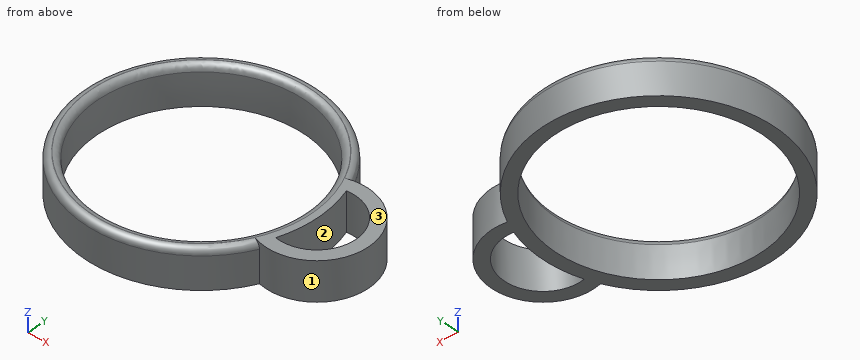
```python
from build123d import *

# Parameters (mm, degrees)
F4_DEPTH = 1.5
F5_DEPTH = 1.5
F6_R     = 0.5


with BuildPart() as f2:
    # F1 (on Front) → F2 (revolve)
    with BuildSketch(Plane.XZ):
        with BuildLine():
            Line((-8.0375234668, 1.5), (-9.0375234668, 1.5))
            Line((-9.0375234668, 1.5), (-9.0375234668, -1.5))
            Line((-9.0375234668, -1.5), (-8.0375234668, -1.5))
            ThreePointArc((-8.0375234668, -1.5), (-8, 0), (-8.0375234668, 1.5))
        make_face()
    revolve(axis=Axis((0, 0, 9.5071946271), (0, 0, 1)))

    # F3 (on Top) → F4 (join)
    with BuildSketch(Plane.XY):
        with BuildLine():
            ThreePointArc((8.5376016897, -2.9641504352), (8.3565039155, -3.4417543091), (8.1487128008, -3.9083641213))
            ThreePointArc((8.1487128008, -3.9083641213), (13, 0), (8.1487128008, 3.9083641213))
            ThreePointArc((8.1487128008, 3.9083641213), (8.3565039155, 3.4417543091), (8.5376016897, 2.9641504352))
            ThreePointArc((8.5376016897, 2.9641504352), (12, 0), (8.5376016897, -2.9641504352))
        make_face()
    extrude(amount=-F4_DEPTH)

    # F5 (add): a face of the model
    f5_faces = [f2.faces().sort_by_distance(p)[0] for p in [
        (8.4430138573, 3.4773847555, 0),
    ]]
    extrude(f5_faces, amount=F5_DEPTH)

    # F6
    f6_edges = [f2.edges().sort_by_distance(p)[0] for p in [
        (-9.037523, 0, 1.5),
        (8.037523, 0, 1.5),
    ]]
    fillet(f6_edges, radius=F6_R)


solid = f2.part
```
Source: CAD feature listing. Evaluate the final solid. Frame: model axes, mm. Face numbers are marked on the shaded views. Round coordinates to 2 decimals unless told otherwise and drop trailing zeros. Loops run counter-clockwise (first coordinate to the right, second up) from the corner with the lowest first, then second, coordinate; pieces in that order, holes last.
(1) Section query C-C (z = -1). Output: boundary loops of the cut face in (x, y).
From the geometry:
outline: (8.15, -3.91) arc R4 ccw (long way) to (8.15, 3.91) arc R9.04 ccw (long way) to start; hole circle Ø16.03 at (0, 0); hole (8.54, -2.96) arc R3 ccw (long way) to (8.54, 2.96) arc R9.04 cw to start
(2) Material intervals for probe 1 along X at (y, z) = (0, 0.35); probe 2 along Y at (x, z) = (-6.25, 0.7); probe 3 along Y at (x, z) = (-4.25, 1.25), sorted ascending.
From the geometry:
probe 1: x = -9.04 to -8, 8 to 9.04, 12 to 13
probe 2: y = -6.53 to -5.01, 5.01 to 6.53
probe 3: y = -7.9 to -6.88, 6.88 to 7.9
(3) Section query A-A (z = 0.5). Output: boundary loops of the cut face in (x, y), and give its area (3 significant figures).
From the geometry:
outline: (8.15, -3.91) arc R4 ccw (long way) to (8.15, 3.91) arc R9.04 ccw (long way) to start; hole circle Ø16.01 at (0, 0); hole (8.54, -2.96) arc R3 ccw (long way) to (8.54, 2.96) arc R9.04 cw to start
area: 67.6 mm2
(4) Contact query for flat-ended pins moving along their axis: pin 1 Ø6 at (x, y) = (4.5, 1) entering from -Z; pin 2 Ø6 at (x, y) = (7, 7) entering from -Z. Output: stop coordinate, or through.
From the geometry:
pin 1: passes through
pin 2: stops at z = -1.5
(5) Pull-direction query (Y, two-part tool) for the marked faces 1, 2 and 3; classes: +Y half, -Y half, draft (parallel to the pull), parting line (faces both ways), or undercut.
From the geometry:
face 1: parting line
face 2: undercut
face 3: draft
(6) Section query B-B (y = -1). Give the number of separate pieces and of enclosed holes in the cut face, and give its area (3 significant figures).
From the geometry:
separate pieces: 3
enclosed holes: 0
area: 9.17 mm2
